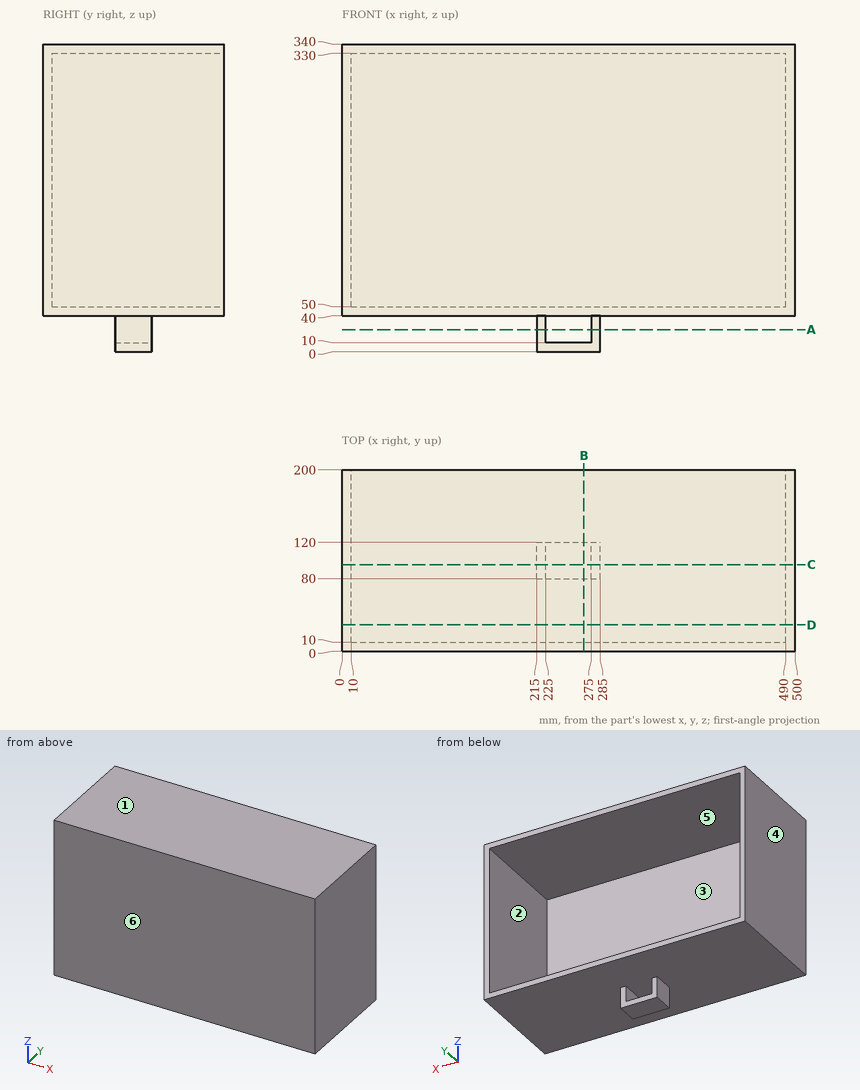
Geometry check sheet. Reference: drawing and pictorial views, mm from the part's lowest x, y, z. A direction names the side the tool comes from. Coordinates: 2 decimals unless noted, no trailing zeros. Write each loop counter-clockwise with the first axis right and the second up, starting at its lowest first coordinate (ties: lowest second). Pieces come first, ordered by that corner, then holes. Notation, with made-up numbers: M 30.5,5.5 L 41.5,5.5 A19 cw 41.5,22.5 Z; hole C 26,42.5 d5. An arc over 180 degrees is marked long. Write item = value, one per line. Start each with the question number.
1. Sectioned sample at B-B (x = 267). Record the cut outline in (y, z).
2. Mould release check, pull along Z, two halves, no side actions. Record for the marked faces 1, 2, 3 and 4: pulls with the +Z half, pulls with the -Z half, needs draft (parallel to the pull), parting line crosses it, or undercut.
3. Sectioned sample at A-A (z = 24.5). Record the cut outline in (x, y), then the cut area to 3 significant figures.
4. Thickness scan on probe 1 along Z at (x, y) = (240, 108); probe 2 along Z at (x, y) = (90, 121.5); probe 3 along X at (y, z) = (184.5, 235). Record the ranges inside material, lowest first.
5. Sectioned sample at C-C (y = 95.5). Record the cut outline in (x, z), then the cut area to 3 significant figures.
6. Go/stop test with flat-tipped pins: pin 1 (3 mm diameter, centred on x = 183.5, y = 59, fed in from -Z); pin 2 (1 mm diameter, centred on y = 151, z = 185, fed in from -X); pin 3 (12 mm diameter, centred on x = 116.5, z = 259, fed in from +Y); pin 4 (24 mm diameter, centred on y = 101, z = 18, fed in from +X). Record where each tip stops, or that it passes through.
7. Sectioned sample at D-D (y = 29). Record the cut outline in (x, z).
8. Tool access check on the marked faces 5 and 6. Record the directions out of +Z, -Z, +X, -X, +Y, -Y that give a thin tool (end or side, any length) a straight path to the whole face; none if there is none.
The answers:
q1.outline = M 0,40 L 200,40 L 200,50 L 10,50 L 10,330 L 200,330 L 200,340 L 0,340 Z; M 80,0 L 120,0 L 120,10 L 80,10 Z
q2.face_1 = pulls with the +Z half
q2.face_2 = undercut
q2.face_3 = undercut
q2.face_4 = needs draft
q3.outline = M 215,80 L 225,80 L 225,120 L 215,120 Z; M 275,80 L 285,80 L 285,120 L 275,120 Z
q3.area = 800 mm²
q4.probe_1 = 0 to 10, 40 to 50, 330 to 340
q4.probe_2 = 40 to 50, 330 to 340
q4.probe_3 = 0 to 10, 490 to 500
q5.outline = M 0,40 L 215,40 L 215,0 L 285,0 L 285,40 L 500,40 L 500,340 L 0,340 Z; hole M 10,50 L 490,50 L 490,330 L 10,330 Z; hole M 225,10 L 275,10 L 275,40 L 225,40 Z
q5.area = 16,900 mm²
q6.pin_1 = 40
q6.pin_2 = 0
q6.pin_3 = 10
q6.pin_4 = 285
q7.outline = M 0,40 L 500,40 L 500,340 L 0,340 Z; hole M 10,50 L 490,50 L 490,330 L 10,330 Z
q8.face_5 = +Y
q8.face_6 = +Z, -Z, +X, -X, -Y
